Geometry: final body of the model. Coordinates: model frame, mm. Face numbers are marked on the shaded views. A direction names the side the tool comes from. Coordinates: 2 decimals unless noted, no trailing zeros. Loops run counter-clockwise (first coordinate to the right, second up) from the corner with the lowest first, then second, coordinate; pieces in that order, holes last. Notation, with made-up numbers: (-18.75, -35.5) - (-13.75, -35.5) arc R36 ccw to (-13.75, 0.5) - close; hole circle Ø9 at (-25, 60). An arc over 180 degrees is marked (long way). Put each result on its own line as item: value. Start each with the question number.
1) Contact query for flat-ended pins moving along their axis: pin 1 Ø3 at (x, y) = (52, 40) entering from +Z; pin 2 Ø6 at (x, z) = (57.5, 4.5) entering from +Y; pin 3 Ø13 at (x, y) = (18, 40) entering from -Z; pin 4 Ø9 at (x, z) = (44, -4) entering from +Y. Output: stop coordinate, or through.
2) Material intervals for line 1 along X through (y, z) = (40, -1.7); line 2 along X through (y, z) = (41, 5); line 3 along Y through (x, z) = (18, 0.85), sorted ascending. Write a range as from..to.
3) Section C-C on y = 18.5. Output: boundary loops of the cut face in (x, z), and give its area (3 significant figures).
4) Section A-A on x = 52. Output: boundary loops of the cut face in (y, z), and give its area (3 significant figures).
5) Draft query along X for the marked faces 1, 2, 3 and 4. Return one class per face: +X half, -X half, draft (parallel to the pull), parting line (faces both ways), or undercut.
6) Section D-D on y = 41. Output: boundary loops of the cut face in (x, z).
7) Reachability of the marked faces 5, 6, 7, 8 and 9 from +Z, -Z, +X, -X, +Y, -Y: full face, straight path, thin tool, end or side. Return the list, or none.
8) Section B-B on z = 9. Output: boundary loops of the cut face in (x, y), and give its area (3 significant figures).
Autodesk Inventor part; units mm, degrees
ref_plane "YZ Plane" through (0, 0, 0) normal (1, 0, 0) x (0, 1, 0)
ref_plane "XZ Plane" through (0, 0, 0) normal (0, 1, 0) x (-1, 0, 0)
ref_plane "XY Plane" through (0, 0, 0) normal (0, 0, 1) x (1, 0, 0)
sketch "Sketch1" plane through (0, 0, 0) normal (0, 0, 1) x (1, 0, 0)
  line L0 (0, 0) -> (70, 0)
  line L1 (70, 0) -> (70, 80)
  line L2 (70, 80) -> (0, 80)
  line L3 (0, 80) -> (0, 0)
  line L4 (12, 80) -> (58, 80)
  line L5 (58, 80) -> (58, 0)
  line L6 (58, 0) -> (12, 0)
  line L7 (12, 0) -> (12, 80)
  point P0 (18, 40)
  point P1 (52, 40)
  point P2 (12, 0)
  dimension "d0" = 70
  dimension "d1" = 80
  dimension "d2" = 34
  dimension "d3" = 18
  dimension "d6" = 40
  dimension "d7" = 40
  dimension "d8" = 12
  dimension "d9" = 12
extrude "Extrusion1" add sketch "Sketch1" against normal blind 6
extrude "Extrusion2" add sketch "Sketch1" along normal blind 10 contours L3 L2 L7 L0 | L5 L2 L1 L0
hole "Hole1" at (18, 40, 0) at (52, 40, 0) direction (0, 0, -1) diameter 4 depth 6
sketch "Sketch2" plane through (0, 0, 0) normal (0, 0, 1) x (1, 0, 0)
  line L0 (12, 0) -> (12, 80)
  line L1 (58, 0) -> (58, 80)
  line L2 (12, 0) -> (58, 0)
  line L3 (58, 0) -> (58, 28)
  line L4 (58, 28) -> (12, 28)
  line L5 (12, 28) -> (12, 0)
  line L6 (58, 80) -> (12, 80)
  line L7 (12, 80) -> (58, 80)
  line L8 (58, 80) -> (58, 52)
  line L9 (58, 52) -> (12, 52)
  line L10 (12, 52) -> (12, 80)
  point P0 (0, 0)
  point P1 (12, 52)
  dimension "d24" = 24
  dimension "d25" = 28
extrude "Extrusion3" cut sketch "Sketch2" against normal blind 6 contours L0 L4 L1 L2 | L0 L6 L1 L9
sketch "Sketch3" plane through (0, 0, 0) normal (0, 0, 1) x (1, 0, 0)
  line L0 (58, 28) -> (12, 28)
  line L1 (12, 52) -> (58, 52)
  line L2 (58, 28) -> (12, 28)
  line L3 (12, 28) -> (12, 52)
  line L4 (12, 52) -> (58, 52)
  line L5 (58, 52) -> (58, 28)
  circle A0 centre (52, 40) radius 2
  circle A1 centre (52, 40) radius 5
  circle A2 centre (18, 40) radius 2
  circle A3 centre (18, 40) radius 5
  point P0 (0, 0)
  dimension "d28" = 10
  dimension "d29" = 10
extrude "Extrusion4" add sketch "Sketch3" along normal blind 2 contours L0 L3 L1 L5
chamfer "Chamfer2" distance 4 angle 45 12 edges at (58, 0, 2) (70, 0, 2) (12, 0, 2) (0, 0, 2) (70, 80, 2) (58, 80, 2) (12, 80, 2) (0, 80, 2) (58, 52, -2) (12, 52, -2) (58, 28, -2) (12, 28, -2)
properties part number "Fan_feet_3DPrint"
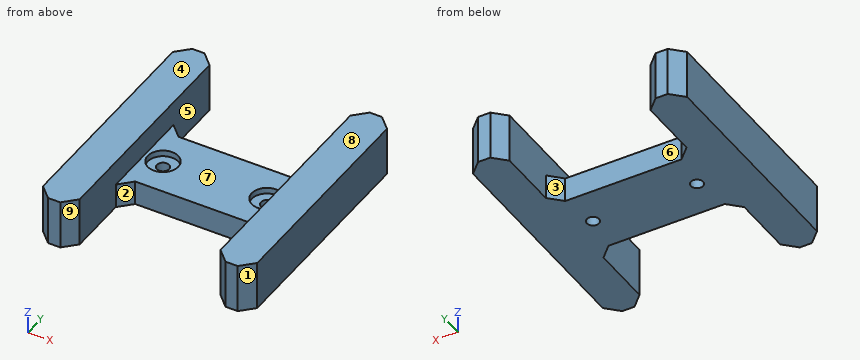
Answer block:
1. pin 1: passes through
1. pin 2: stops at y = 78.5
1. pin 3: stops at z = -6
1. pin 4: stops at y = 52
2. line 1: x = 0..16, 20..50, 54..70
2. line 2: x = 0..12, 58..70
2. line 3: y = 28..35, 45..52
3. outline: (0, -6) - (12, -6) - (12, 10) - (0, 10) - close; (58, -6) - (70, -6) - (70, 10) - (58, 10) - close
3. area: 384 mm²
4. outline: (28, -6) - (38, -6) - (38, 0) - (35, 0) - (35, 2) - (28, 2) - close; (42, -6) - (52, -6) - (52, 2) - (45, 2) - (45, 0) - (42, 0) - close
4. area: 148 mm²
5. face 1: +X half
5. face 2: undercut
5. face 3: undercut
5. face 4: draft
6. outline: (0, -6) - (16.27, -6) - (16.27, 0) - (13.1, 0) - (13.1, 2) - (12, 2) - (12, 10) - (0, 10) - close; (19.73, -6) - (50.27, -6) - (50.27, 0) - (47.1, 0) - (47.1, 2) - (22.9, 2) - (22.9, 0) - (19.73, 0) - close; (53.73, -6) - (70, -6) - (70, 10) - (58, 10) - (58, 2) - (56.9, 2) - (56.9, 0) - (53.73, 0) - close
7. face 5: +Z
7. face 6: +Z, -Z, +Y
7. face 7: +Z, +Y, -Y
7. face 8: +Z, +X, -X, +Y, -Y
7. face 9: +Z, -Z, -Y
8. outline: (0, 4) - (4, 0) - (8, 0) - (12, 4) - (12, 76) - (8, 80) - (4, 80) - (0, 76) - close; (58, 4) - (62, 0) - (66, 0) - (70, 4) - (70, 76) - (66, 80) - (62, 80) - (58, 76) - close
8. area: 1,860 mm²
